from build123d import *

# Parameters (mm, degrees)
F1_DEPTH = 31.75


with BuildPart() as f1:
    # F0 (on Front) → F1 (new body)
    with BuildSketch(Plane.XZ):
        with BuildLine():
            Line((-30.705059, -47.546379), (30.705059, -47.546379))
            Line((30.705059, -47.546379), (30.705059, 47.546379))
            Line((30.705059, 47.546379), (30.629403, 47.546379))
            Line((30.629403, 47.546379), (13.019142, 47.546379))
            ThreePointArc((13.019142, 47.546379), (0, 34.527237), (-13.019142, 47.546379))
            Line((-13.019142, 47.546379), (-30.629403, 47.546379))
            Line((-30.629403, 47.546379), (-30.705059, 47.546379))
            Line((-30.705059, 47.546379), (-30.705059, -47.546379))
        make_face()
        with BuildLine():
            Line((13.019142, 47.546379), (30.629403, 47.546379))
            ThreePointArc((30.629403, 47.546379), (0, 78.175783), (-30.629403, 47.546379))
            Line((-30.629403, 47.546379), (-13.019142, 47.546379))
            ThreePointArc((-13.019142, 47.546379), (0, 60.565521), (13.019142, 47.546379))
        make_face()
    extrude(amount=F1_DEPTH)


solid = f1.part
Check sheet for the modelled part. Datum: model origin and axes. Units: mm. Round coordinates to 2 decimals unless told otherwise and drop trailing zeros. Order: outer loops, then holes, each group sorted by start corner. A loop starts at its lowest first (then second) coordinate and runs counter-clockwise, first axis right, second up.
(1) Cross-section at C-C, the plane z = 49. Enter the section's corners in (x, y), and give its area (3 significant figures).
(2) Cross-section at B-B, the plane y = -2.5. Enter the section's corners in (x, z).
(3) Cross-section at D-D, the plane x = 26.5. Enter the section's corners in (y, z), and give its area (3 significant figures).
(4) Scan lines: probe 1 along Z at (x, y) = (0, -13.5); probe 2 along X at (y, z) = (-16, 53.5); probe 3 along X at (y, z) = (-5, 56). Record each from-to range of solid material in increasing order.
(5) Cross-section at A-A, the plane x = 0. Enter the section's corners in (y, z), and give its area (3 significant figures).
(6) Draft check along Z on faces 1 (the cylindrical face through (1.695, -15.653, 60.455)), 2 (the flat face through (-30.705, -16, 1)), 3 (the cylindrical face through (0.67, -15.65, 78.17)). Enter one of: pulls with the +Z half, pulls with the -Z half, needs draft (parallel to the pull), parting line crosses it, or undercut.
Check sheet entries:
1. outline: (-30.59, -31.75) - (-12.94, -31.75) - (-12.94, 0) - (-30.59, 0) - close; (12.94, -31.75) - (30.59, -31.75) - (30.59, 0) - (12.94, 0) - close
1. area: 1,120 mm2
2. outline: (-30.71, -47.55) - (30.71, -47.55) - (30.71, 47.55) - (30.63, 47.55) arc R30.63 ccw to (-30.63, 47.55) - (-30.71, 47.55) - close; hole circle Ø26.04 at (0, 47.55)
3. outline: (-31.75, -47.55) - (0, -47.55) - (0, 62.91) - (-31.75, 62.91) - close
3. area: 3,510 mm2
4. probe 1: z = -47.55 to 34.53, 60.57 to 78.18
4. probe 2: x = -30.05 to -11.58, 11.58 to 30.05
4. probe 3: x = -29.44 to -9.9, 9.9 to 29.44
5. outline: (-31.75, -47.55) - (0, -47.55) - (0, 34.53) - (-31.75, 34.53) - close; (-31.75, 60.57) - (0, 60.57) - (0, 78.18) - (-31.75, 78.18) - close
5. area: 3,160 mm2
6. face 1: undercut
6. face 2: needs draft
6. face 3: pulls with the +Z half
